Source: three-view drawing plus pictorial views. Frame: mm from the lowest corner of the part. A direction names the side the tool comes from. Give positions to 0.01 mm unless a question says otherwise; leave off trailing zeros. Order: outer loops, then holes, each group sorted by start corner. A loop starts at its lowest first (then second) coordinate and runs counter-clockwise, first axis right, second up. Notation, with made-up numbers: (38.5, 39.25) -> (72.5, 39.25) arc R17 cw to (72.5, 68.25) -> close; hole circle Ø9 at (63, 50). An arc over 180 degrees is marked (long way). Answer in a Markdown table with one row per item.
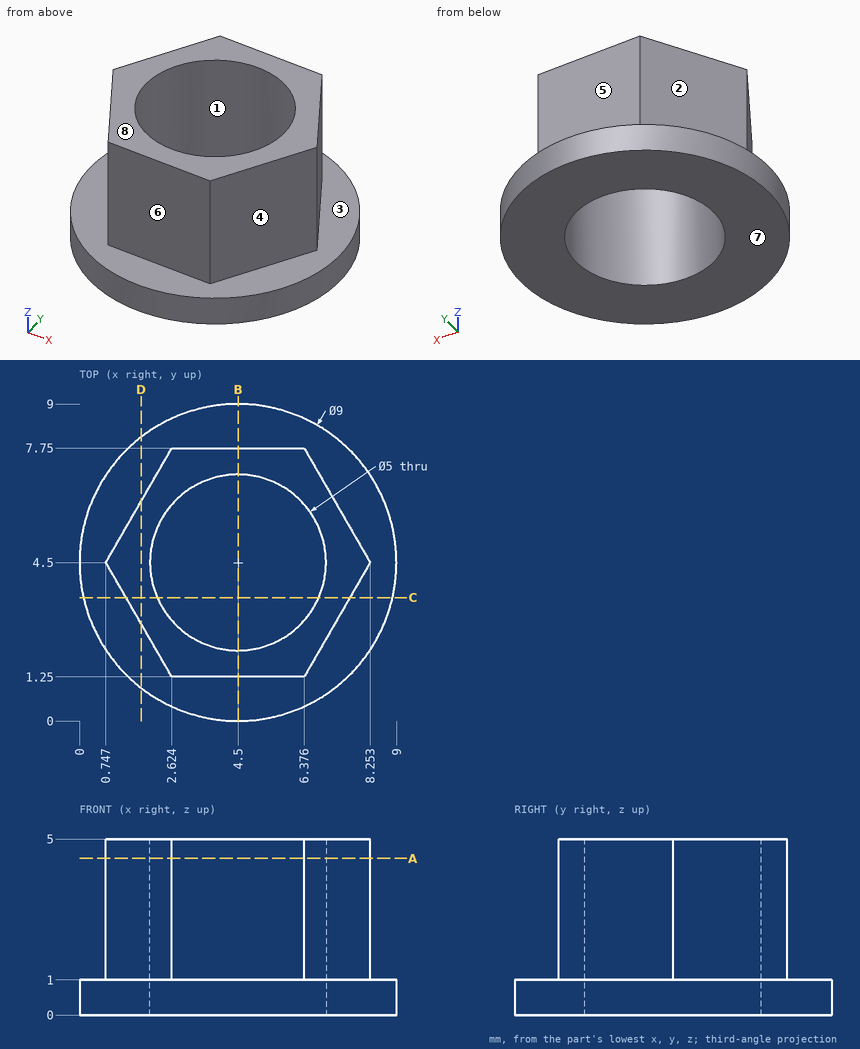
(1) Ray query, probe 1 along Y at (x, z) = (4.5, 3.95); probe 2 along Z at (x, y) = (2.5, 8); probe 3 along X at (y, z) = (6.5, 2.4). Return the intervals inside material, ascending.
A:
| item | result |
|---|---|
| probe 1 | y = 1.25 to 2, 7 to 7.75 |
| probe 2 | z = 0 to 1 |
| probe 3 | x = 1.9 to 3, 6 to 7.1 |
(2) Section query D-D (x = 1.75). Return the cut outline in (y, z), plus the area to 3 significant figures.
A:
| item | result |
|---|---|
| outline | (0.94, 0) -> (8.06, 0) -> (8.06, 1) -> (6.24, 1) -> (6.24, 5) -> (2.76, 5) -> (2.76, 1) -> (0.94, 1) -> close |
| area | 21.0 mm^2 |
(3) Section query B-B (x = 4.5). Return the cut outline in (y, z), plus the area to 3 significant figures.
A:
| item | result |
|---|---|
| outline | (0, 0) -> (2, 0) -> (2, 5) -> (1.25, 5) -> (1.25, 1) -> (0, 1) -> close; (7, 0) -> (9, 0) -> (9, 1) -> (7.75, 1) -> (7.75, 5) -> (7, 5) -> close |
| area | 10.0 mm^2 |
(4) Section query C-C (y = 3.5). Return the cut outline in (x, z) (1 decimal).
A:
| item | result |
|---|---|
| outline | (0.1, 0) -> (2.2, 0) -> (2.2, 5) -> (1.3, 5) -> (1.3, 1) -> (0.1, 1) -> close; (6.8, 0) -> (8.9, 0) -> (8.9, 1) -> (7.7, 1) -> (7.7, 5) -> (6.8, 5) -> close |
(5) Access query for the marked faces 4, 5, 6, 7 and 8. Directions: +Z, -Z, +X, -X, +Y, -Y. A direction counts if a zero-diameter tool reaches every point of the face in a straight line with its end or side. Return the directions, or none.
A:
| item | result |
|---|---|
| face 4 | +Z, +X, -Y |
| face 5 | +Z, +X, -X, +Y |
| face 6 | +Z, +X, -X, -Y |
| face 7 | -Z, +X, -X, +Y, -Y |
| face 8 | +Z, +X, -X, +Y, -Y |
(6) Section query A-A (z = 4.45). Return the cut outline in (x, y).
A:
| item | result |
|---|---|
| outline | (0.75, 4.5) -> (2.62, 1.25) -> (6.38, 1.25) -> (8.25, 4.5) -> (6.38, 7.75) -> (2.62, 7.75) -> close; hole circle Ø5 at (4.5, 4.5) |
(7) First-contact query: pin 1 Ø1.5 at (x, z) = (6, 3.5) entering from -Y. Flat tip, straight axial feed; report the tip coordinate or a pass-through.
A:
| item | result |
|---|---|
| pin 1 | stops at y = 1.25 |
(8) Pull-direction query (X, two-part tool) for the marked faces 1, 2 and 3; classes: +X half, -X half, draft (parallel to the pull), parting line (faces both ways), or undercut.
A:
| item | result |
|---|---|
| face 1 | undercut |
| face 2 | -X half |
| face 3 | draft |
